Geometry check sheet. Reference: the model listing, model coordinates, mm. A direction names the side the tool comes from. Coordinates: 2 decimals unless noted, no trailing zeros. Answer as a JSON object with one key per item and string values. Group by question number.
```python
from build123d import *

# Parameters (mm, degrees)
SKETCH1_W           = 1695.45
SKETCH1_H           = 184.15
BOSS_EXTRUDE1_DEPTH = 38.1
CHAMFER1_SIZE       = 2.54
CHAMFER2_SIZE       = 2.54
SKETCH2_R           = 19.05
CUT_EXTRUDE1_DEPTH  = 3.175


with BuildPart() as part:
    # Sketch1 → Boss-Extrude1 (new body)
    with BuildSketch(Plane(origin=(0, 0, 0), x_dir=(1, 0, 0), z_dir=(0, 1, 0))):
        with Locations((847.725, 92.075)):
            Rectangle(SKETCH1_W, SKETCH1_H)
        with BuildLine():
            Line((1240.0153, 110.16615), (1181.2651, 110.16615))
            ThreePointArc((1181.2651, 110.16615), (1168.5651, 122.86615), (1181.2651, 135.56615))
            Line((1181.2651, 135.56615), (1240.0153, 135.56615))
            ThreePointArc((1240.0153, 135.56615), (1252.7153, 122.86615), (1240.0153, 110.16615))
        make_face(mode=Mode.SUBTRACT)
        with BuildLine():
            Line((254, 110.31855), (312.7502, 110.31855))
            ThreePointArc((312.7502, 110.31855), (325.4502, 97.61855), (312.7502, 84.91855))
            Line((312.7502, 84.91855), (254, 84.91855))
            ThreePointArc((254, 84.91855), (241.3, 97.61855), (254, 110.31855))
        make_face(mode=Mode.SUBTRACT)
    extrude(amount=BOSS_EXTRUDE1_DEPTH)

    # Chamfer1
    chamfer1_edges = [part.edges().sort_by_distance(p)[0] for p in [
        (1695.45, 38.1, -92.075),
        (1252.7153, 38.1, -122.86615),
        (847.725, 38.1, -184.15),
        (1210.6402, 38.1, -135.56615),
        (1168.5651, 38.1, -122.86615),
        (1210.6402, 38.1, -110.16615),
        (325.4502, 38.1, -97.61855),
        (283.3751, 38.1, -110.31855),
        (241.3, 38.1, -97.61855),
        (283.3751, 38.1, -84.91855),
        (0, 38.1, -92.075),
        (847.725, 38.1, 0),
    ]]
    chamfer(chamfer1_edges, length=CHAMFER1_SIZE)

    # Chamfer2
    chamfer2_edges = [part.edges().sort_by_distance(p)[0] for p in [
        (1252.7153, 0, -122.86615),
        (1210.6402, 0, -135.56615),
        (1168.5651, 0, -122.86615),
        (1210.6402, 0, -110.16615),
        (325.4502, 0, -97.61855),
        (283.3751, 0, -110.31855),
        (241.3, 0, -97.61855),
        (283.3751, 0, -84.91855),
        (847.725, 0, -184.15),
        (1695.45, 0, -92.075),
        (847.725, 0, 0),
        (0, 0, -92.075),
    ]]
    chamfer(chamfer2_edges, length=CHAMFER2_SIZE)

    # Sketch2 → Cut-Extrude1 (cut)
    with BuildSketch(Plane(origin=(0, 0, 0), x_dir=(1, 0, 0), z_dir=(0, 1, 0))):
        with Locations((283.3751, 97.61855)):
            Circle(SKETCH2_R)
        with Locations((1210.6402, 122.86615)):
            Circle(SKETCH2_R)
    extrude(amount=CUT_EXTRUDE1_DEPTH, mode=Mode.SUBTRACT)


solid = part.part
```
1) Go/stop test with a flat-tipped pin: pin 1 Ø5 at (x, z) = (283.5, -81.5) entering from -Y (3 decimals). Record where the tip stops, or that it passes through.
2) Material ranges on probe 1 along X at (y, z) = (26, -96); probe 2 along Z at (x, y) = (1236.5, 12); probe 3 along X at (y, z) = (32, -132), recorded low to high. Write a range as [from, to].
3) Set-up check for faces 1 (the flat face through (1211, 19, -110.166)), 2 (the flat face through (836, 0, -93)): record each of +Z, -Z, +X, -X, +Y, -Y from which the full face is reachable in a straight line by a thin tool's end or side.
4) Draft check along Z on faces 3 (the flat face through (836, 19, 0)), 4 (the flat face through (283, 19, -110.319)), 5 (the flat face through (1210, 19, -135.566)), 6 (the flat face through (0, 19, -91)). Enter one of: +Z half, -Z half, draft (parallel to the pull), parting line (faces both ways), or undercut.
Entries:
{
 "1": {"pin 1": "y = 3.175"},
 "2": {"probe 1": "[0, 241.4], [325.35, 1695.45]", "probe 2": "[-184.15, -135.57], [-110.17, 0]", "probe 3": "[0, 1172.44], [1248.84, 1695.45]"},
 "3": {"face 1": "+Y, -Y", "face 2": "+Z, -Z, +X, -X, -Y"},
 "4": {"face 3": "+Z half", "face 4": "undercut", "face 5": "undercut", "face 6": "draft"}
}
